Source: CAD feature listing. Evaluate the final solid. Frame: model axes, mm. Round coordinates to 2 decimals unless told otherwise and drop trailing zeros. Write each loop counter-clockwise with the first axis right and the second up, starting at its lowest first coordinate (ties: lowest second). Pieces come first, ordered by that corner, then holes. Notation, with made-up numbers: M 0,43 L 30,43 A13 ccw 30,66 Z; hole C 35.5,72.25 d3. An arc over 180 degrees is marked long. Use a Markdown table: item, result.
```python
from build123d import *

# Parameters (mm, degrees)
SKETCH1_W           = 210
SKETCH1_H           = 120
BOSS_EXTRUDE1_DEPTH = 5
CUT_EXTRUDE1_DEPTH  = 2
SKETCH3_R           = 1.5
CUT_EXTRUDE3_DEPTH  = 5
SKETCH4_R           = 6
CUT_EXTRUDE4_DEPTH  = 5
SKETCH5_R           = 1.5
CUT_EXTRUDE5_DEPTH  = 10


with BuildPart() as part:
    # Sketch1 → Boss-Extrude1 (new body)
    with BuildSketch(Plane.XY):
        with Locations((105, -60)):
            Rectangle(SKETCH1_W, SKETCH1_H)
    extrude(amount=BOSS_EXTRUDE1_DEPTH)

    # Sketch2 → Cut-Extrude1 (cut)
    with BuildSketch(Plane.XY.offset(5)):
        with BuildLine():
            ThreePointArc((125, -60), (105, -40), (85, -60))
            Line((85, -60), (125, -60))
        make_face()
        with BuildLine():
            Line((125, -60), (85, -60))
            ThreePointArc((85, -60), (105, -80), (125, -60))
        make_face()
    extrude(amount=-CUT_EXTRUDE1_DEPTH, mode=Mode.SUBTRACT)

    # Sketch3 → Cut-Extrude3 (cut)
    with BuildSketch(Plane.XY.offset(3)):
        with Locations((105, -45)):
            Circle(SKETCH3_R)
        with Locations((120, -60)):
            Circle(SKETCH3_R)
        with Locations((105, -75)):
            Circle(SKETCH3_R)
        with Locations((90, -60)):
            Circle(SKETCH3_R)
    extrude(amount=-CUT_EXTRUDE3_DEPTH, mode=Mode.SUBTRACT)

    # Sketch4 → Cut-Extrude4 (cut)
    with BuildSketch(Plane.XY.offset(3)):
        with Locations((105, -60)):
            Circle(SKETCH4_R)
    extrude(amount=-CUT_EXTRUDE4_DEPTH, mode=Mode.SUBTRACT)

    # Sketch5 → Cut-Extrude5 (cut)
    with BuildSketch(Plane.XY.offset(5)):
        with Locations((45, -115)):
            Circle(SKETCH5_R)
        with Locations((105, -115)):
            Circle(SKETCH5_R)
        with Locations((165, -115)):
            Circle(SKETCH5_R)
    extrude(amount=-CUT_EXTRUDE5_DEPTH, mode=Mode.SUBTRACT)


solid = part.part
```
Q1. Line query: L1, parallel to Y at x = 105, z = 1.45; L2, parallel to X at y = -115, z = 1.5; L3, parallel to Y at x = 120, z = 1.6. Output: solid intervals per line, ascending.
Results are:
| item | result |
|---|---|
| L1 | -120 to -116.5, -113.5 to -76.5, -73.5 to -66, -54 to -46.5, -43.5 to 0 |
| L2 | 0 to 43.5, 46.5 to 103.5, 106.5 to 163.5, 166.5 to 210 |
| L3 | -120 to -61.5, -58.5 to 0 |
Q2. First-contact query: pin 1 Ø5 at (x, y) = (105, -75) entering from +Z; pin 2 Ø3.5 at (x, y) = (45, -115) entering from +Z; pin 3 Ø11 at (x, y) = (105, -60) entering from -Z. Flat tips, straight axial feed; report the tip coordinate or a pass-through.
Results are:
| item | result |
|---|---|
| pin 1 | z = 3 |
| pin 2 | z = 5 |
| pin 3 | through |
Q3. Section B-B on y = -50. Return loops of the section in (x, z), plus the area to 3 significant figures.
Results are:
| item | result |
|---|---|
| outline | M 0,0 L 210,0 L 210,5 L 122.32,5 L 122.32,3 L 87.68,3 L 87.68,5 L 0,5 Z |
| area | 981 mm^2 |
Q4. Section A-A on z = 4.2. Return loops of the section in (x, y), plus the area to 3 significant figures.
Results are:
| item | result |
|---|---|
| outline | M 0,-120 L 210,-120 L 210,0 L 0,0 Z; hole C 45,-115 d3; hole C 105,-60 d40; hole C 105,-115 d3; hole C 165,-115 d3 |
| area | 23,900 mm^2 |
Q5. Mould query, pull axis X, two halves, no side actions, for faces 1 (the flat face through (100, -64, 3)), 2 (the cylindrical face through (121, -48, 4)), 3 (the flat face through (210, -61, 2)), 4 (the flat face through (127, -59, 5)). Classes: +X half, -X half, draft (parallel to the pull), parting line (faces both ways), or undercut.
Results are:
| item | result |
|---|---|
| face 1 | undercut |
| face 2 | undercut |
| face 3 | +X half |
| face 4 | draft |
